from build123d import *

# Parameters (mm, degrees)
SKETCH1_R           = 2.5
BOSS_EXTRUDE1_DEPTH = 12
SKETCH2_R           = 3
CUT_EXTRUDE1_DEPTH  = 25


with BuildPart() as part:
    # Sketch1 → Boss-Extrude1 (new body)
    with BuildSketch(Plane(origin=(0, 0, 0), x_dir=(0, 0, -1), z_dir=(1, 0, 0))):
        with BuildLine():
            Line((-45, 0), (-45, 30))
            Line((-45, 30), (45, 30))
            Line((45, 30), (45, 0))
            ThreePointArc((45, 0), (0, -45), (-45, 0))
        make_face()
        with Locations((-15, 0)):
            Circle(SKETCH1_R, mode=Mode.SUBTRACT)
        with Locations((15, 0)):
            Circle(SKETCH1_R, mode=Mode.SUBTRACT)
    extrude(amount=BOSS_EXTRUDE1_DEPTH)

    # Sketch2 → Cut-Extrude1 (cut)
    with BuildSketch(Plane(origin=(0, 30, 0), x_dir=(1, 0, 0), z_dir=(0, 1, 0))):
        with Locations((6, 40.5)):
            Circle(SKETCH2_R)
        with Locations((6, 7.5)):
            Circle(SKETCH2_R)
        with Locations((6, -7.5)):
            Circle(SKETCH2_R)
        with Locations((6, -40.5)):
            Circle(SKETCH2_R)
    extrude(amount=-CUT_EXTRUDE1_DEPTH, mode=Mode.SUBTRACT)


solid = part.part
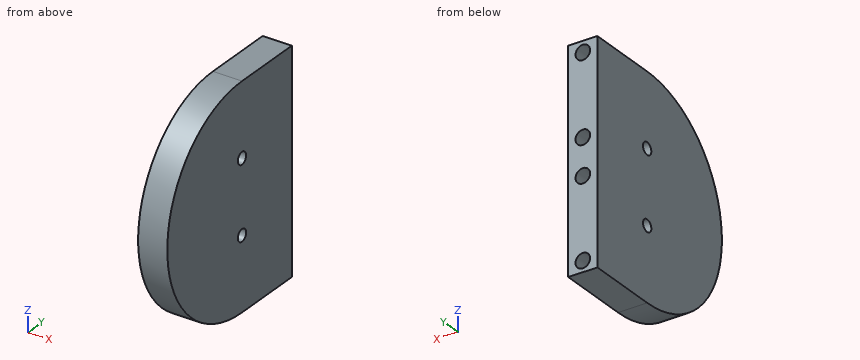
Geometry: final body of the model. Coordinates: model frame, mm. Give positions to 0.01 mm unless a question says otherwise; leave off trailing zeros. Loops run counter-clockwise (first coordinate to the right, second up) from the corner with the lowest first, then second, coordinate; pieces in that order, holes last. Notation, with made-up numbers: (51.25, 26.5) -> (63.25, 26.5) arc R16 cw to (63.25, 45.5) -> close; hole circle Ø3 at (-34.75, 34.25). An arc over 180 degrees is marked (long way). Put each result on its own line as item: value.
1. Ray query, line 1 along Z through (x, y) = (6, 21.75); line 2 along Z through (x, y) = (5.25, 1); line 3 along Z through (x, y) = (8.5, 19). Return the intervals inside material, ascending. Write a range as [from, to].
Taken from the geometry:
line 1: z = [-45, -43.5], [-37.5, -10.5], [-4.5, 4.5], [10.5, 37.5], [43.5, 45]
line 2: z = [-45, -17.29], [-12.71, 12.71], [17.29, 45]
line 3: z = [-45, -42.16], [-38.84, -9.16], [-5.84, 5.84], [9.16, 38.84], [42.16, 45]
2. Pin query (flat end, axial travel): P1, Ø5, axis at x = 5.5, z = -19.5, coming from the -Y side; P2, Ø5.5, axis at x = 6, z = -7.5, coming from the -Y side; P3, Ø1.8, axis at x = 5.5, z = 41.5, coming from the +Y side. Return the tip coordinate at first contact, or that it passes through.
Taken from the geometry:
P1: stops at y = -41.67
P2: stops at y = -44.75
P3: stops at y = 5
3. Cut plane A-A (x = 6). Return the cut outline in (y, z), plus the area to 3 significant figures.
Taken from the geometry:
outline: (0, -45) -> (30, -45) -> (30, -43.5) -> (5, -43.5) -> (5, -37.5) -> (30, -37.5) -> (30, -10.5) -> (5, -10.5) -> (5, -4.5) -> (30, -4.5) -> (30, 4.5) -> (5, 4.5) -> (5, 10.5) -> (30, 10.5) -> (30, 37.5) -> (5, 37.5) -> (5, 43.5) -> (30, 43.5) -> (30, 45) -> (0, 45) arc R45 ccw to start; hole circle Ø5 at (0, -15); hole circle Ø5 at (0, 15)
area: 5,240 mm2
4. Cut plane D-D (y = -39). Return the cut outline in (x, z).
Taken from the geometry:
outline: (0, -22.45) -> (12, -22.45) -> (12, 22.45) -> (0, 22.45) -> close
5. Cut plane B-B (z = -14). Return the cut outline in (x, y).
Taken from the geometry:
outline: (0, -42.77) -> (12, -42.77) -> (12, -2.29) -> (0, -2.29) -> close; (0, 2.29) -> (12, 2.29) -> (12, 30) -> (0, 30) -> close
6. Cut plane C-C (z = 7.5). Return the cut outline in (x, y).
Taken from the geometry:
outline: (0, -44.37) -> (12, -44.37) -> (12, 30) -> (9, 30) -> (9, 5) -> (3, 5) -> (3, 30) -> (0, 30) -> close
